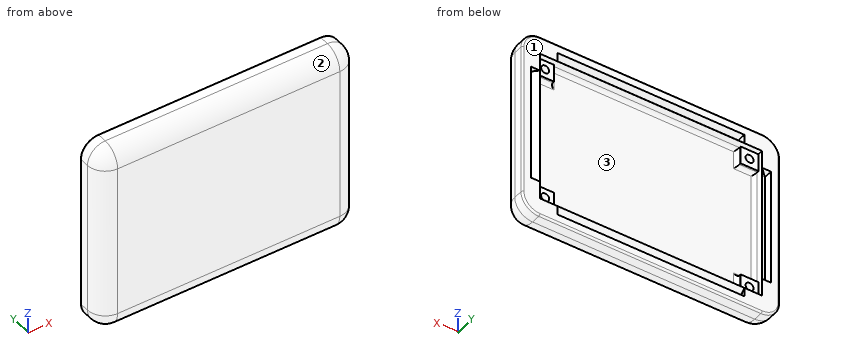
```python
from build123d import *

# Parameters (mm, degrees)
SKETCH1_W               = 145
SKETCH1_H               = 106
BOSS_EXTRUDE1_DEPTH     = 16
CUT_EXTRUDE1_START      = 16
SKETCH1_4_W             = 125
SKETCH1_4_H             = 86
CUT_EXTRUDE1_DEPTH      = 6
CUT_EXTRUDE3_DEPTH      = 52.5
CUT_EXTRUDE4_DEPTH      = 33
FILLET1_R               = 10
SKETCH5_W               = 10
SKETCH5_H               = 10
BOSS_EXTRUDE3_DEPTH     = 3
MIRROR6_COPY_1_SKETCH_W = 10
MIRROR6_COPY_1_SKETCH_H = 10
MIRROR6_COPY_1_DEPTH    = 3
FILLET3_R               = 2
FILLET11_R              = 1


with BuildPart() as part:
    # Sketch1 → Boss-Extrude1 (new body)
    with BuildSketch(Plane(origin=(0, 0, 0), x_dir=(1, 0, 0), z_dir=(0, 1, 0))):
        Rectangle(SKETCH1_W, SKETCH1_H)
    extrude(amount=BOSS_EXTRUDE1_DEPTH)

    # Sketch1<4> → Cut-Extrude1 (cut)
    with BuildSketch(Plane(origin=(0, 0, 0), x_dir=(1, 0, 0), z_dir=(0, 1, 0)).offset(CUT_EXTRUDE1_START)):
        Rectangle(SKETCH1_4_W, SKETCH1_4_H)
    extrude(amount=-CUT_EXTRUDE1_DEPTH, mode=Mode.SUBTRACT)

    # Sketch3 → Cut-Extrude3 (cut, symmetric)
    with BuildSketch(Plane(origin=(0, 0, 0), x_dir=(0, 0, -1), z_dir=(1, 0, 0))):
        Polygon((-48, 16), (-43, 16), (-48, 11), align=None)
    cut_extrude3 = extrude(amount=CUT_EXTRUDE3_DEPTH, both=True, mode=Mode.SUBTRACT)

    # Sketch4 → Cut-Extrude4 (cut, symmetric)
    with BuildSketch(Plane.XY):
        Polygon((-62.5, 16), (-67.5, 16), (-67.5, 11), align=None)
    cut_extrude4 = extrude(amount=CUT_EXTRUDE4_DEPTH, both=True, mode=Mode.SUBTRACT)

    # Mirror1: Cut-Extrude4 across plane
    add(cut_extrude4.mirror(Plane(origin=(0, 0, 0), x_dir=(0, 0, 1), z_dir=(1, 0, 0))), mode=Mode.SUBTRACT)

    # Mirror4: Cut-Extrude3 across plane
    add(cut_extrude3.mirror(Plane.XY), mode=Mode.SUBTRACT)

    # Fillet1
    fillet1_edges = [part.edges().sort_by_distance(p)[0] for p in [
        (0, 0, -53),
        (72.5, 0, 0),
        (0, 0, 53),
        (-72.5, 0, 0),
        (-72.5, 8, -53),
        (72.5, 8, -53),
        (72.5, 8, 53),
        (-72.5, 8, 53),
    ]]
    fillet(fillet1_edges, radius=FILLET1_R)

    # Sketch5 → Boss-Extrude3 (add)
    with BuildSketch(Plane(origin=(0, 10, 0), x_dir=(1, 0, 0), z_dir=(0, 1, 0))):
        with Locations((-57.5, 38)):
            Rectangle(SKETCH5_W, SKETCH5_H)
    boss_extrude3 = extrude(amount=BOSS_EXTRUDE3_DEPTH)

    # Sketch7 → M4 Clearance Hole1 (revolve, cut)
    with BuildSketch(Plane(origin=(-57.5, 13, -38), x_dir=(0, 0, 1), z_dir=(1, 0, 0))):
        Polygon((0, 0), (0, 7.25), (2.25, 5), (2.25, 0), align=None)
    m4_clearance_hole1 = revolve(axis=Axis((-57.5, 19.35, -38), (0, -1, 0)), mode=Mode.SUBTRACT)

    # Mirror5: Boss-Extrude3, M4 Clearance Hole1 across plane
    add(boss_extrude3.mirror(Plane.XY))
    add(m4_clearance_hole1.mirror(Plane.XY), mode=Mode.SUBTRACT)

    # Mirror6: Boss-Extrude3, M4 Clearance Hole1 across plane
    add(boss_extrude3.mirror(Plane(origin=(0, 0, 0), x_dir=(0, 0, 1), z_dir=(1, 0, 0))))
    add(m4_clearance_hole1.mirror(Plane(origin=(0, 0, 0), x_dir=(0, 0, 1), z_dir=(1, 0, 0))), mode=Mode.SUBTRACT)

    # Mirror6 copy 1 sketch → Mirror6 copy 1 (add)
    with BuildSketch(Plane(origin=(0, 10, 0), x_dir=(-1, 0, 0), z_dir=(0, 1, 0))):
        with Locations((-57.5, 38)):
            Rectangle(MIRROR6_COPY_1_SKETCH_W, MIRROR6_COPY_1_SKETCH_H)
    extrude(amount=MIRROR6_COPY_1_DEPTH)

    # Mirror6 copy 2 sketch → Mirror6 copy 2 (revolve, cut)
    with BuildSketch(Plane(origin=(57.5, 13, 38), x_dir=(0, 0, -1), z_dir=(-1, 0, 0))):
        Polygon((0, 0), (0, 7.25), (2.25, 5), (2.25, 0), align=None)
    revolve(axis=Axis((57.5, 19.35, 38), (0, -1, 0)), mode=Mode.SUBTRACT)

    # Fillet3
    fillet3_edges = [part.edges().sort_by_distance(p)[0] for p in [
        (-52.5, 10, -38),
        (-57.5, 10, -33),
        (-62.5, 10, 0),
        (-57.5, 10, 33),
        (-52.5, 10, 38),
        (0, 10, -43),
        (57.5, 10, -33),
        (52.5, 10, -38),
        (0, 10, 43),
        (62.5, 10, 0),
        (52.5, 10, 38),
        (57.5, 10, 33),
    ]]
    fillet(fillet3_edges, radius=FILLET3_R)

    # Fillet11
    fillet11_edges = [part.edges().sort_by_distance(p)[0] for p in [
        (0, 16, 53),
        (72.5, 16, 0),
        (0, 16, -53),
        (-72.5, 16, 0),
        (-69.571067812, 16, 50.071067812),
        (69.571067812, 16, 50.071067812),
        (69.571067812, 16, -50.071067812),
        (-69.571067812, 16, -50.071067812),
    ]]
    fillet(fillet11_edges, radius=FILLET11_R)


solid = part.part
```
Design review of the part built by this model. Coordinates are the model's own, in mm. Face numbers are marked on the shaded views. Round coordinates to 2 decimals unless told otherwise and drop trailing zeros. Write each loop counter-clockwise with the first axis right and the second up, starting at its lowest first coordinate (ties: lowest second). Pieces come first, ordered by that corner, then holes.
Item 1: We need section C-C on y = 4.25. Write out the cut boundary in (x, z).
Item 2: We need section A-A on x = -41.5. Write out the cut boundary in (y, z), and give its area (3 significant figures).
Item 3: Clearance check with flat-ended pins moving along their axes: pin 1 Ø8 at (y, z) = (6.5, 9.5) entering from -X; pin 2 Ø5 at (x, z) = (-57.5, 38) entering from +Y; pin 3 Ø2 at (x, z) = (42, -4) entering from +Y; pin 4 Ø2.5 at (x, y) = (-64, 13) entering from +Z. State where each tip first meets the part, or that it passes through.
Item 4: The part is to be moulded in two halves that separate along Z. For the marked faces 1, 2 and 3, say which applies: +Z half, -Z half, draft (parallel to the pull), parting line (faces both ways), or undercut.
Item 5: We need section B-B on z = 19.5. Write out the cut boundary in (x, y).
Item 6: For probe 1 along X at (y, z) = (10.65, -38); probe 2 along Z at (x, y) = (-57.5, 9.65); probe 3 along Z at (x, y) = (-57.5, 10.65), list the stretches that pass through material, from the lowest coordinate up.
Returned:
1. outline: (-70.68, -43) arc R8.18 ccw to (-62.5, -51.18) - (62.5, -51.18) arc R8.18 ccw to (70.68, -43) - (70.68, 43) arc R8.18 ccw to (62.5, 51.18) - (-62.5, 51.18) arc R8.18 ccw to (-70.68, 43) - close
2. outline: (0, -43) arc R10 ccw to (10, -53) - (15, -53) arc R1 ccw to (16, -52) - (16, -48) - (11, -48) - (16, -43) - (12, -43) arc R2 cw to (10, -41) - (10, 41) arc R2 cw to (12, 43) - (16, 43) - (11, 48) - (16, 48) - (16, 52) arc R1 ccw to (15, 53) - (10, 53) arc R10 ccw to (0, 43) - close
2. area: 1,110 mm2
3. pin 1: stops at x = -72.5
3. pin 2: stops at y = 13
3. pin 3: stops at y = 10
3. pin 4: stops at z = 53
4. face 1: draft
4. face 2: +Z half
4. face 3: undercut
5. outline: (-72.5, 10) arc R10 ccw to (-62.5, 0) - (62.5, 0) arc R10 ccw to (72.5, 10) - (72.5, 15) arc R1 ccw to (71.5, 16) - (67.5, 16) - (67.5, 11) - (62.5, 16) - (62.5, 12) arc R2 cw to (60.5, 10) - (-60.5, 10) arc R2 cw to (-62.5, 12) - (-62.5, 16) - (-67.5, 11) - (-67.5, 16) - (-71.5, 16) arc R1 ccw to (-72.5, 15) - close
6. probe 1: x = -72.5 to -59.75, -55.25 to -51.98, 51.98 to 55.25, 59.75 to 72.5
6. probe 2: z = -52.99 to -40.25, -35.75 to 35.75, 40.25 to 52.99
6. probe 3: z = -53 to -40.25, -35.75 to -32.48, 32.48 to 35.75, 40.25 to 53
